Design review of the part built by this model. Coordinates are the model's own, in mm. A direction names the side the tool comes from. Coordinates: 2 decimals unless noted, no trailing zeros. Loops run counter-clockwise (first coordinate to the right, second up) from the corner with the lowest first, then second, coordinate; pieces in that order, holes last. Notation, with made-up numbers: (46.25, 75.5) - (76.25, 75.5) arc R10 cw to (76.25, 85.5) - close; hole circle Ø3 at (2, 14.25). An arc over 180 degrees is marked (long way). Use one line per item in the form item = value. Start each with the question number.
(1) Add section A-A (z = 10.75). State the section outline as (x, y) points, plus the area to 3 significant figures.
(2) Add section B-B (x = -76). State the section outline as (y, z) points.
(3) Tool access review of faces 4 (the face through (-105, -60, 8)), 5 (the face through (-107, 4, 8)), 6 (the face through (102, 4, 8)): name each direction out of +Z, -Z, +X, -X, +Y, -Y from which nothing blocks a thin tool from reaching the whole face with its end or side.
(4) For L1, parallel to X at y = 67, z = 1.1; L2, parallel to Y at x = 0, z = 2.05; L3, parallel to X at y = 24.5, z = 6.5, list the stretches that pass through material, from the lowest coordinate up.
(5) Clearance check with flat-ended pins moving along their axes: pin 1 Ø3 at (x, y) = (0, -67) entering from -Z; pin 2 Ø10 at (x, y) = (21.5, 3) entering from +Z; pin 3 Ø3 at (y, z) = (-56, 7) entering from -X; pin 4 Ø1.5 at (x, z) = (-104, 8) entering from -Y. State where each tip first meets the part, or that it passes through.
(6) Add section D-D (x = 18.5). State the section outline as (y, z) points, plus the area to 3 significant figures.
(7) Add section C-C (y = -39). State the section outline as (x, z) points, plus the area to 3 significant figures.
(8) The part is to be moulded in two halves that separate along X. For faces 1 (the face through (104, 6, 13)), 2 (the face through (-102, 4, 8)), 3 (the face through (107, 4, 8)), say which applies: pulls with the +X half, pulls with the -X half, needs draft (parallel to the pull), parting line crosses it, or undercut.
```python
from build123d import *

# Parameters (mm, degrees)
SKETCH_W     = 228
SKETCH_H     = 140
SKETCH_R     = 1.75
PAD_DEPTH    = 3
SKETCH001_W  = 5
SKETCH001_H  = 130
PAD001_DEPTH = 13
SKETCH002_R  = 1.15
POCKET_DEPTH = 112.5


with BuildPart() as part:
    # Sketch → Pad (new body)
    with BuildSketch(Plane.XY):
        with Locations((4, 0)):
            Rectangle(SKETCH_W, SKETCH_H)
        with Locations((-90, 67)):
            Circle(SKETCH_R, mode=Mode.SUBTRACT)
        with Locations((0, 67)):
            Circle(SKETCH_R, mode=Mode.SUBTRACT)
        with Locations((90, 67)):
            Circle(SKETCH_R, mode=Mode.SUBTRACT)
        with Locations((-90, -67)):
            Circle(SKETCH_R, mode=Mode.SUBTRACT)
        with Locations((0, -67)):
            Circle(SKETCH_R, mode=Mode.SUBTRACT)
        with Locations((90, -67)):
            Circle(SKETCH_R, mode=Mode.SUBTRACT)
        with BuildLine():
            ThreePointArc((-90, 43.5), (-91.75, 41.75), (-90, 40))
            Line((-90, 40), (-10, 40))
            ThreePointArc((-10, 40), (-8.25, 41.75), (-10, 43.5))
            Line((-90, 43.5), (-10, 43.5))
        make_face(mode=Mode.SUBTRACT)
        with BuildLine():
            ThreePointArc((-90, 33.5), (-91.75, 31.75), (-90, 30))
            Line((-90, 30), (-10, 30))
            ThreePointArc((-10, 30), (-8.25, 31.75), (-10, 33.5))
            Line((-90, 33.5), (-10, 33.5))
        make_face(mode=Mode.SUBTRACT)
        with BuildLine():
            ThreePointArc((-90, 23.5), (-91.75, 21.75), (-90, 20))
            Line((-90, 20), (-10, 20))
            ThreePointArc((-10, 20), (-8.25, 21.75), (-10, 23.5))
            Line((-90, 23.5), (-10, 23.5))
        make_face(mode=Mode.SUBTRACT)
        with BuildLine():
            ThreePointArc((-90, 13.5), (-91.75, 11.75), (-90, 10))
            Line((-90, 10), (-10, 10))
            ThreePointArc((-10, 10), (-8.25, 11.75), (-10, 13.5))
            Line((-90, 13.5), (-10, 13.5))
        make_face(mode=Mode.SUBTRACT)
        with BuildLine():
            ThreePointArc((-90, 3.5), (-91.75, 1.75), (-90, 0))
            Line((-90, 0), (-10, 0))
            ThreePointArc((-10, 0), (-8.25, 1.75), (-10, 3.5))
            Line((-90, 3.5), (-10, 3.5))
        make_face(mode=Mode.SUBTRACT)
    extrude(amount=PAD_DEPTH)

    # Sketch001 → Pad001 (join)
    with BuildSketch(Plane.XY):
        with Locations((104.5, 5)):
            Rectangle(SKETCH001_W, SKETCH001_H)
        with Locations((-104.5, 5)):
            Rectangle(SKETCH001_W, SKETCH001_H)
    extrude(amount=PAD001_DEPTH)

    # Sketch002 → Pocket (cut, symmetric)
    with BuildSketch(Plane.YZ):
        with Locations((-56, 7)):
            Circle(SKETCH002_R)
        with Locations((66, 7)):
            Circle(SKETCH002_R)
    extrude(amount=POCKET_DEPTH, both=True, mode=Mode.SUBTRACT)


solid = part.part
```
Computed values:
q1.outline = (-107, -60) - (-102, -60) - (-102, 70) - (-107, 70) - close; (102, -60) - (107, -60) - (107, 70) - (102, 70) - close
q1.area = 1,300 mm^2
q2.outline = (-70, 0) - (0, 0) - (0, 3) - (-70, 3) - close; (3.5, 0) - (10, 0) - (10, 3) - (3.5, 3) - close; (13.5, 0) - (20, 0) - (20, 3) - (13.5, 3) - close; (23.5, 0) - (30, 0) - (30, 3) - (23.5, 3) - close; (33.5, 0) - (40, 0) - (40, 3) - (33.5, 3) - close; (43.5, 0) - (70, 0) - (70, 3) - (43.5, 3) - close
q3.face_4 = +Z, +X, -X, -Y
q3.face_5 = +Z, -X, +Y, -Y
q3.face_6 = +Z, +Y, -Y
q4.L1 = -110 to -91.75, -88.25 to -1.75, 1.75 to 88.25, 91.75 to 118
q4.L2 = -70 to -68.75, -65.25 to 65.25, 68.75 to 70
q4.L3 = -107 to -102, 102 to 107
q5.pin_1 = through
q5.pin_2 = 3
q5.pin_3 = -107
q5.pin_4 = -60
q6.outline = (-70, 0) - (70, 0) - (70, 3) - (-70, 3) - close
q6.area = 420 mm^2
q7.outline = (-110, 0) - (118, 0) - (118, 3) - (107, 3) - (107, 13) - (102, 13) - (102, 3) - (-102, 3) - (-102, 13) - (-107, 13) - (-107, 3) - (-110, 3) - close
q7.area = 784 mm^2
q8.face_1 = needs draft
q8.face_2 = undercut
q8.face_3 = pulls with the +X half
